```python
from build123d import *

# Parameters (mm, degrees)
SKETCH1_W           = 120
SKETCH1_H           = 120
BOSS_EXTRUDE1_DEPTH = 2
FILLET1_R           = 5
FILLET2_R           = 5
FILLET3_R           = 5
FILLET4_R           = 5
SKETCH2_W           = 20
SKETCH2_H           = 20
CUT_EXTRUDE1_DEPTH  = 10
FILLET5_R           = 2
FILLET6_R           = 2
SKETCH4_R           = 1.5
CUT_EXTRUDE2_DEPTH  = 10


with BuildPart() as part:
    # Sketch1 → Boss-Extrude1 (new body)
    with BuildSketch(Plane(origin=(0, 0, 0), x_dir=(1, 0, 0), z_dir=(0, 1, 0))):
        Rectangle(SKETCH1_W, SKETCH1_H)
    extrude(amount=BOSS_EXTRUDE1_DEPTH)

    # Fillet1
    fillet1_edges = [part.edges().sort_by_distance(p)[0] for p in [
        (60, 1, 60),
    ]]
    fillet(fillet1_edges, radius=FILLET1_R)

    # Fillet2
    fillet2_edges = [part.edges().sort_by_distance(p)[0] for p in [
        (-60, 1, 60),
    ]]
    fillet(fillet2_edges, radius=FILLET2_R)

    # Fillet3
    fillet3_edges = [part.edges().sort_by_distance(p)[0] for p in [
        (60, 1, -60),
    ]]
    fillet(fillet3_edges, radius=FILLET3_R)

    # Fillet4
    fillet4_edges = [part.edges().sort_by_distance(p)[0] for p in [
        (-60, 1, -60),
    ]]
    fillet(fillet4_edges, radius=FILLET4_R)

    # Sketch2 → Cut-Extrude1 (cut)
    with BuildSketch(Plane(origin=(0, 2, 0), x_dir=(1, 0, 0), z_dir=(0, 1, 0))):
        Polygon((-47.5, -47.5), (-17.5, -17.5), (-17.5, 17.5), (-47.5, 47.5), align=None)
        Polygon((18, -30), (-18, -30), (-32.5, -44.5), (32.5, -44.5), align=None)
        Rectangle(SKETCH2_W, SKETCH2_H)
        Polygon((35.5, 47.5), (-35.5, 47.5), (-18, 30), (18, 30), align=None)
        Polygon((17.5, -17.5), (47.5, -47.5), (47.5, 47.5), (17.5, 17.5), align=None)
    extrude(amount=-CUT_EXTRUDE1_DEPTH, mode=Mode.SUBTRACT)

    # Fillet5
    fillet5_edges = [part.edges().sort_by_distance(p)[0] for p in [
        (-35.5, 1, -47.5),
        (35.5, 1, -47.5),
    ]]
    fillet(fillet5_edges, radius=FILLET5_R)

    # Fillet6
    fillet6_edges = [part.edges().sort_by_distance(p)[0] for p in [
        (-18, 1, -30),
        (18, 1, -30),
        (-32.5, 1, 44.5),
        (-18, 1, 30),
        (18, 1, 30),
        (32.5, 1, 44.5),
        (10, 1, 10),
        (-10, 1, 10),
        (-10, 1, -10),
        (10, 1, -10),
        (-17.5, 1, -17.5),
        (-17.5, 1, 17.5),
        (-47.5, 1, 47.5),
        (-47.5, 1, -47.5),
        (47.5, 1, -47.5),
        (47.5, 1, 47.5),
        (17.5, 1, 17.5),
        (17.5, 1, -17.5),
    ]]
    fillet(fillet6_edges, radius=FILLET6_R)

    # Sketch4 → Cut-Extrude2 (cut)
    with BuildSketch(Plane.XZ):
        with Locations(Location((-36.293024341, -48.5, 0), (0, 0, 270))):
            Circle(SKETCH4_R)
        with Locations(Location((-31.293024341, 48.5, 0), (0, 0, 270))):
            Circle(SKETCH4_R)
        with Locations(Location((31.293024341, 48.5, 0), (0, 0, 270))):
            Circle(SKETCH4_R)
        with Locations(Location((36.293024341, -48.5, 0), (0, 0, 270))):
            Circle(SKETCH4_R)
    extrude(amount=-CUT_EXTRUDE2_DEPTH, mode=Mode.SUBTRACT)


solid = part.part
```
The model under review builds one solid part; all positions refer to its coordinate system, in mm. A direction names the side the tool comes from. Round coordinates to 2 decimals unless told otherwise and drop trailing zeros. Write each loop counter-clockwise with the first axis right and the second up, starting at its lowest first coordinate (ties: lowest second). Pieces come first, ordered by that corner, then holes. Notation, with made-up numbers: M 29,13 L 53,13 A11 cw 53,34 Z; hole C -19.5,32 d9. An arc over 180 degrees is marked long. Use CSV: the item, a comma, the result in double quotes. Start each with the question number.
(1) We need section D-D, the plane z = 48.5. State the section outline as (x, y) points, then the cut area to 3 significant figures.
(2) Tool access review of faces 4 (the face through (31, 1, -31)), 5 (the face through (12, 2, -1)): name each direction out of +Z, -Z, +X, -X, +Y, -Y from which nothing blocks a thin tool from reaching the whole face with its end or side.
(3) We need section C-C, the plane z = -39.5. State the section outline as (x, y) points.
(4) We need section B-B, the plane x = 0. State the section outline as (y, z) points.
(5) For line 1 along X through (y, z) = (1.45, -48.5); line 2 along Z through (x, y) = (-3, 1.05); line 3 along X through (y, z) = (0.65, 11), list the stretches that pass through material, from the lowest coordinate up.
(6) We need section A-A, the plane z = -21. State the section outline as (x, y) points.
(7) The part is to be moulded in two halves that separate along X. For faces 1 (the face through (59, 1, -58)), 2 (the face through (-25, 1, -37)), 3 (the face through (-58, 1, 59)), say which applies: +X half, -X half, draft (parallel to the pull), parting line (faces both ways), or undercut.
(8) Clearance check with a flat-ended pin moving along its axis: P1, Ø4, axis at x = 22, z = -21, coming from the -Y side. State where the tip first meets the part, or that it passes through.
Findings:
1,outline,"M -60,0 L -32.79,0 L -32.79,2 L -60,2 Z; M -29.79,0 L 29.79,0 L 29.79,2 L -29.79,2 Z; M 32.79,0 L 60,0 L 60,2 L 32.79,2 Z"
1,area,"228 mm^2"
2,face 4,"+Y, -Y"
2,face 5,"+Z, -Z, +X, -X, +Y"
3,outline,"M -60,0 L -47.5,0 L -47.5,2 L -60,2 Z; M -39.5,0 L -27.5,0 L -27.5,2 L -39.5,2 Z; M 27.5,0 L 39.5,0 L 39.5,2 L 27.5,2 Z; M 47.5,0 L 60,0 L 60,2 L 47.5,2 Z"
4,outline,"M 0,-60 L 2,-60 L 2,-47.5 L 0,-47.5 Z; M 0,-30 L 2,-30 L 2,-10 L 0,-10 Z; M 0,10 L 2,10 L 2,30 L 0,30 Z; M 0,44.5 L 2,44.5 L 2,60 L 0,60 Z"
5,line 1,"-60 to -37.79, -34.79 to 34.79, 37.79 to 60"
5,line 2,"-60 to -47.5, -30 to -10, 10 to 30, 44.5 to 60"
5,line 3,"-60 to -47.5, -17.5 to 17.5, 47.5 to 60"
6,outline,"M -60,0 L -47.5,0 L -47.5,2 L -60,2 Z; M -21,0 L 21,0 L 21,2 L -21,2 Z; M 47.5,0 L 60,0 L 60,2 L 47.5,2 Z"
7,face 1,"+X half"
7,face 2,"undercut"
7,face 3,"-X half"
8,P1,"y = 0"
